Source: CAD feature listing. Evaluate the final solid. Frame: model axes, mm. Coordinates: 2 decimals unless noted, no trailing zeros. Write each loop counter-clockwise with the first axis right and the second up, starting at its lowest first coordinate (ties: lowest second). Pieces come first, ordered by that corner, then holes. Notation, with made-up numbers: (47, 43.25) - (103, 43.25) arc R17 cw to (103, 50.25) - close; hole circle Ø9 at (53.5, 38.5). An arc over 180 degrees is marked (long way). One line per question, with ' | ' between items. Start each with the question number.
Q1. Draft query along Z for faces 1 (the face through (95.31, 0.78, -102)), 2 (the face through (90.53, 0.8, -91.27)), 3 (the face through (49, 1.588, -51)). Return one class per face: +Z half, -Z half, draft (parallel to the pull), parting line (faces both ways), or undercut.
Q2. Cut plane C-C, the plane y = 0.55. Give the number of separate pieces and of enclosed holes in the cut face, plus the area to 3 significant figures.
Q3. Cut plane A-A, the plane z = -50. Return loops of the section in (x, y).
Q4. Contact query for flat-ended pins moving along their axis: P1, Ø3.5, axis at x = 10, z = -90, coming from the +Y side; P2, Ø0.5, axis at y = 1, z = -66.5, coming from the +X side; P3, Ø2, axis at x = 10, z = -64, coming from the +Y side; P4, Ø0.8, axis at y = 0.5, z = -56.5, coming from the +X side. Output: stop coordinate, or through.
Q5. Line query: line 1 (Z direction, x = 8.5, y = 0.15); line 2 (X direction, y = 0.3, z = -65.5); line 3 (X direction, y = 0.6, z = -20.5). Output: solid intervals per line, ascending.
Q6. Cut plane D-D, the plane x = 54. Return loops of the section in (y, z), plus the area to 3 significant figures.
Q7. Cut plane B-B, the plane x = 37.5. Return loops of the section in (y, z), plus the area to 3 significant figures.
```python
from build123d import *

# Parameters (mm, degrees)
BOSS_EXTRUDE1_DEPTH       = 1.5875
CUT_EXTRUDE1_DEPTH        = 5
SKETCH4_R                 = 1.375
CUT_EXTRUDE2_DEPTH        = 5
CUT_EXTRUDE4_DEPTH        = 5
CUT_EXTRUDE6_DEPTH        = 5
CIRPATTERN1_COUNT         = 4
CIRPATTERN4_COUNT         = 4
F_2_5MM_DOWEL_HOLE1_D     = 2.6
F_2_5MM_DOWEL_HOLE2_D     = 2.6
F_9_0_9_DIAMETER_HOLE1_D  = 9
CIRPATTERN5_COUNT         = 4
FILLET1_R                 = 2
F_2_5MM_DOWEL_HOLE3_D     = 3.3
F_2_5MM_DOWEL_SLOT1_DEPTH = 1.5875
SKETCH19_W                = 24
SKETCH19_H                = 34
CUT_EXTRUDE7_DEPTH        = 10
FILLET2_R                 = 2
FILLET3_R                 = 1


# Read off the part's stored shape, not the designer's step: Ø2.5mm Dowel Slot1
with BuildPart() as part:
    # Sketch2 → Boss-Extrude1 (new body)
    with BuildSketch(Plane(origin=(0, 0, 0), x_dir=(1, 0, 0), z_dir=(0, 1, 0))):
        Polygon((30, 0), (88, 0), (88, -9), (100, -9), (100, 0), (100, 100), (100, 109), (88, 109), (88, 100), (30, 100), (30, 109), (0, 109), (0, 100), (0, 0), (0, -9), (30, -9), align=None)
    extrude(amount=BOSS_EXTRUDE1_DEPTH)

    # Sketch3 → Cut-Extrude1 (cut)
    with BuildSketch(Plane(origin=(0, 1.5875, 0), x_dir=(1, 0, 0), z_dir=(0, 1, 0))):
        with BuildLine():
            Line((11.25, 80), (11.25, 20))
            ThreePointArc((11.25, 20), (10, 18.75), (8.75, 20))
            Line((8.75, 20), (8.75, 80))
            ThreePointArc((8.75, 80), (10, 81.25), (11.25, 80))
        make_face()
    extrude(amount=-CUT_EXTRUDE1_DEPTH, mode=Mode.SUBTRACT)

    # Sketch4 → Cut-Extrude2 (cut)
    with BuildSketch(Plane(origin=(0, 1.5875, 0), x_dir=(1, 0, 0), z_dir=(0, 1, 0))):
        with Locations(Location((10, 10, 0), (0, 0, 270))):
            Circle(SKETCH4_R)
    cut_extrude2 = extrude(amount=-CUT_EXTRUDE2_DEPTH, mode=Mode.SUBTRACT)

    # Sketch6 → Cut-Extrude4 (cut)
    with BuildSketch(Plane(origin=(0, 1.5875, 0), x_dir=(1, 0, 0), z_dir=(0, 1, 0))):
        with BuildLine():
            Line((49.25, 11.25), (50.75, 11.25))
            ThreePointArc((50.75, 11.25), (52, 10), (50.75, 8.75))
            Line((50.75, 8.75), (49.25, 8.75))
            ThreePointArc((49.25, 8.75), (48, 10), (49.25, 11.25))
        make_face()
    cut_extrude4 = extrude(amount=-CUT_EXTRUDE4_DEPTH, mode=Mode.SUBTRACT)

    # Sketch8 → Cut-Extrude6 (cut)
    with BuildSketch(Plane(origin=(0, 1.5875, 0), x_dir=(1, 0, 0), z_dir=(0, 1, 0))):
        with BuildLine():
            Line((30, 51.65), (40, 51.65))
            ThreePointArc((40, 51.65), (41.65, 50), (40, 48.35))
            Line((40, 48.35), (30, 48.35))
            ThreePointArc((30, 48.35), (28.35, 50), (30, 51.65))
        make_face()
    cut_extrude6 = extrude(amount=-CUT_EXTRUDE6_DEPTH, mode=Mode.SUBTRACT)

    # CirPattern1: Cut-Extrude6 ×4 about axis
    cirpattern1_axis = Axis((50, 0, -50), (0, 1, 0))
    for i in range(1, CIRPATTERN1_COUNT):
        add(cut_extrude6.rotate(cirpattern1_axis, i * 360 / CIRPATTERN1_COUNT), mode=Mode.SUBTRACT)

    # CirPattern4: Cut-Extrude2 ×4 about axis
    cirpattern4_axis = Axis((50, 0, -50), (0, 1, 0))
    for i in range(1, CIRPATTERN4_COUNT):
        add(cut_extrude2.rotate(cirpattern4_axis, i * 360 / CIRPATTERN4_COUNT), mode=Mode.SUBTRACT)

    # Mirror6: Cut-Extrude4 across plane
    add(cut_extrude4.mirror(Plane(origin=(0, 0, -50), x_dir=(1, 0, 0), z_dir=(0, 0, -1))), mode=Mode.SUBTRACT)

    # Ø2.5mm Dowel Hole1 (through all)
    with Locations(Plane(origin=(0, 1.5875, 0), x_dir=(1, 0, 0), z_dir=(0, 1, 0))):
        with Locations((62.5, 15), (37.5, 15)):
            Hole(F_2_5MM_DOWEL_HOLE1_D / 2)

    # Ø2.5mm Dowel Hole2 (through all)
    with Locations(Plane(origin=(0, 1.5875, 0), x_dir=(1, 0, 0), z_dir=(0, 1, 0))):
        with Locations((42.7, 59.4), (67.7, 59.4)):
            Hole(F_2_5MM_DOWEL_HOLE2_D / 2)

    # Ø9.0 (9) Diameter Hole1 (through all)
    with Locations(Plane(origin=(0, 1.5875, 0), x_dir=(1, 0, 0), z_dir=(0, 1, 0))):
        with Locations((80, 20)):
            f_9_0_9_diameter_hole1 = Hole(F_9_0_9_DIAMETER_HOLE1_D / 2)

    # CirPattern5: Ø9.0 (9) Diameter Hole1 ×4 about axis
    cirpattern5_axis = Axis((50, 0, -50), (0, 1, 0))
    for i in range(1, CIRPATTERN5_COUNT):
        add(f_9_0_9_diameter_hole1.rotate(cirpattern5_axis, i * 360 / CIRPATTERN5_COUNT), mode=Mode.SUBTRACT)

    # Fillet1
    fillet1_edges = [part.edges().sort_by_distance(p)[0] for p in [
        (30, 0.79375, 0),
        (30, 0.79375, 9),
        (0, 0.79375, 9),
        (0, 0.79375, -109),
        (30, 0.79375, -109),
        (30, 0.79375, -100),
        (88, 0.79375, -100),
        (88, 0.79375, -109),
        (100, 0.79375, -109),
        (100, 0.79375, 9),
        (88, 0.79375, 9),
        (88, 0.79375, 0),
    ]]
    fillet(fillet1_edges, radius=FILLET1_R)

    # Ø2.5mm Dowel Hole3 (through all)
    with Locations(Plane(origin=(0, 1.5875, 0), x_dir=(1, 0, 0), z_dir=(0, 1, 0))):
        with Locations((94, -3), (94, 103)):
            Hole(F_2_5MM_DOWEL_HOLE3_D / 2)

    # Ø2.5mm Dowel Slot1 outline → Ø2.5mm Dowel Slot1 (cut)
    with BuildSketch(Plane(origin=(0, 0, 0), x_dir=(1, 0, 0), z_dir=(0, 1, 0))):
        with BuildLine():
            Line((6.65, 101.35), (23.35, 101.35))
            ThreePointArc((23.35, 101.35), (25, 103), (23.35, 104.65))
            Line((23.35, 104.65), (6.65, 104.65))
            ThreePointArc((6.65, 104.65), (5, 103), (6.65, 101.35))
        make_face()
        with BuildLine():
            Line((6.65, -4.65), (23.35, -4.65))
            ThreePointArc((23.35, -4.65), (25, -3), (23.35, -1.35))
            Line((23.35, -1.35), (6.65, -1.35))
            ThreePointArc((6.65, -1.35), (5, -3), (6.65, -4.65))
        make_face()
    extrude(amount=F_2_5MM_DOWEL_SLOT1_DEPTH, mode=Mode.SUBTRACT)

    # Sketch19 → Cut-Extrude7 (cut)
    with BuildSketch(Plane(origin=(0, 1.5875, 0), x_dir=(1, 0, 0), z_dir=(0, 1, 0))):
        with Locations((88, 50)):
            Rectangle(SKETCH19_W, SKETCH19_H)
    extrude(amount=-CUT_EXTRUDE7_DEPTH, mode=Mode.SUBTRACT)

    # Fillet2
    fillet2_edges = [part.edges().sort_by_distance(p)[0] for p in [
        (100, 0.79375, -67),
        (100, 0.79375, -33),
    ]]
    fillet(fillet2_edges, radius=FILLET2_R)

    # Fillet3
    fillet3_edges = [part.edges().sort_by_distance(p)[0] for p in [
        (76, 0.79375, -33),
        (76, 0.79375, -67),
    ]]
    fillet(fillet3_edges, radius=FILLET3_R)


solid = part.part
```
Reply:
1) face 1: undercut | face 2: undercut | face 3: draft
2) separate pieces: 1 | enclosed holes: 23 | area: 9,150 mm^2
3) outline: (0, 0) - (8.75, 0) - (8.75, 1.59) - (0, 1.59) - close; (11.25, 0) - (28.35, 0) - (28.35, 1.59) - (11.25, 1.59) - close; (41.65, 0) - (58.35, 0) - (58.35, 1.59) - (41.65, 1.59) - close; (71.65, 0) - (76, 0) - (76, 1.59) - (71.65, 1.59) - close
4) P1: stops at y = 1.59 | P2: stops at x = 76.34 | P3: passes through | P4: stops at x = 76
5) line 1: z = -109 to -104.65, -101.35 to 1.35, 4.65 to 9 | line 2: x = 0 to 8.75, 11.25 to 48.35, 51.65 to 76 | line 3: x = 0 to 8.75, 11.25 to 15.53, 24.47 to 75.53, 84.47 to 100
6) outline: (0, -100) - (1.59, -100) - (1.59, 0) - (0, 0) - close | area: 159 mm^2
7) outline: (0, -100) - (1.59, -100) - (1.59, -51.65) - (0, -51.65) - close; (0, -48.35) - (1.59, -48.35) - (1.59, -16.3) - (0, -16.3) - close; (0, -13.7) - (1.59, -13.7) - (1.59, 0) - (0, 0) - close | area: 149 mm^2
